```python
from build123d import *

# Parameters (mm, degrees)
F1_DEPTH = 91.42907
F2_R     = 7.5
F3_DEPTH = 2
F4_DEPTH = 5.7
F5_R     = 5
F6_DEPTH = 25
F6_TAPER = 13
F7_SIZE  = 0.5


with BuildPart() as f1:
    # F0 (on Top) → F1 (new body)
    with BuildSketch(Plane.XY):
        Polygon((1, 6.5773502692), (-1, 6.5773502692), (-1, 0.5773502692), (-6.1961524227, -2.4226497308), (-5.1961524227, -4.1547005384), (0, -1.1547005384), (5.1961524227, -4.1547005384), (6.1961524227, -2.4226497308), (1, 0.5773502692), align=None)
    extrude(amount=F1_DEPTH)

    # F2 (on face) → F3 (join)
    with BuildSketch(Plane.XY.offset(91.42907)):
        Circle(F2_R)
        with BuildLine():
            ThreePointArc((1, 5.941432908), (4.6003056964, 3.8907341852), (6.025, 0))
            ThreePointArc((6.025, 0), (5.9293486908, -1.0693217956), (5.6454318332, -2.1046910502))
            Line((5.6454318332, -2.1046910502), (6.1961524227, -2.4226497308))
            Line((6.1961524227, -2.4226497308), (5.1961524227, -4.1547005384))
            Line((5.1961524227, -4.1547005384), (4.6454318332, -3.8367418578))
            ThreePointArc((4.6454318332, -3.8367418578), (0, -6.025), (-4.6454318332, -3.8367418578))
            Line((-4.6454318332, -3.8367418578), (-5.1961524227, -4.1547005384))
            Line((-5.1961524227, -4.1547005384), (-6.1961524227, -2.4226497308))
            Line((-6.1961524227, -2.4226497308), (-5.6454318332, -2.1046910502))
            ThreePointArc((-5.6454318332, -2.1046910502), (-5.2178030578, 3.0125), (-1, 5.941432908))
            Line((-1, 5.941432908), (-1, 6.5773502692))
            Line((-1, 6.5773502692), (1, 6.5773502692))
            Line((1, 6.5773502692), (1, 5.941432908))
        make_face(mode=Mode.SUBTRACT)
        with BuildLine():
            Line((1, 0.5773502692), (1, 5.941432908))
            ThreePointArc((1, 5.941432908), (0, 6.025), (-1, 5.941432908))
            Line((-1, 5.941432908), (-1, 0.5773502692))
            Line((-1, 0.5773502692), (-5.6454318332, -2.1046910502))
            ThreePointArc((-5.6454318332, -2.1046910502), (-5.2178030578, -3.0125), (-4.6454318332, -3.8367418578))
            Line((-4.6454318332, -3.8367418578), (0, -1.1547005384))
            Line((0, -1.1547005384), (4.6454318332, -3.8367418578))
            ThreePointArc((4.6454318332, -3.8367418578), (5.2178030578, -3.0125), (5.6454318332, -2.1046910502))
            Line((5.6454318332, -2.1046910502), (1, 0.5773502692))
        make_face()
        with BuildLine():
            ThreePointArc((5.6454318332, -2.1046910502), (5.9293486908, -1.0693217956), (6.025, 0))
            ThreePointArc((6.025, 0), (4.6003056964, 3.8907341852), (1, 5.941432908))
            Line((1, 5.941432908), (1, 0.5773502692))
            Line((1, 0.5773502692), (5.6454318332, -2.1046910502))
        make_face()
        with BuildLine():
            ThreePointArc((-4.6454318332, -3.8367418578), (0, -6.025), (4.6454318332, -3.8367418578))
            Line((4.6454318332, -3.8367418578), (0, -1.1547005384))
            Line((0, -1.1547005384), (-4.6454318332, -3.8367418578))
        make_face()
        with BuildLine():
            Line((-1, 0.5773502692), (-1, 5.941432908))
            ThreePointArc((-1, 5.941432908), (-5.2178030578, 3.0125), (-5.6454318332, -2.1046910502))
            Line((-5.6454318332, -2.1046910502), (-1, 0.5773502692))
        make_face()
        with BuildLine():
            ThreePointArc((-4.6454318332, -3.8367418578), (-5.2178030578, -3.0125), (-5.6454318332, -2.1046910502))
            Line((-5.6454318332, -2.1046910502), (-6.1961524227, -2.4226497308))
            Line((-6.1961524227, -2.4226497308), (-5.1961524227, -4.1547005384))
            Line((-5.1961524227, -4.1547005384), (-4.6454318332, -3.8367418578))
        make_face()
        with BuildLine():
            Line((6.1961524227, -2.4226497308), (5.6454318332, -2.1046910502))
            ThreePointArc((5.6454318332, -2.1046910502), (5.2178030578, -3.0125), (4.6454318332, -3.8367418578))
            Line((4.6454318332, -3.8367418578), (5.1961524227, -4.1547005384))
            Line((5.1961524227, -4.1547005384), (6.1961524227, -2.4226497308))
        make_face()
        with BuildLine():
            ThreePointArc((-1, 5.941432908), (0, 6.025), (1, 5.941432908))
            Line((1, 5.941432908), (1, 6.5773502692))
            Line((1, 6.5773502692), (-1, 6.5773502692))
            Line((-1, 6.5773502692), (-1, 5.941432908))
        make_face()
    extrude(amount=F3_DEPTH)

    # F2 (on face) → F4 (join)
    with BuildSketch(Plane.XY.offset(91.42907)):
        Circle(F2_R)
        with BuildLine():
            ThreePointArc((1, 5.941432908), (4.6003056964, 3.8907341852), (6.025, 0))
            ThreePointArc((6.025, 0), (5.9293486908, -1.0693217956), (5.6454318332, -2.1046910502))
            Line((5.6454318332, -2.1046910502), (6.1961524227, -2.4226497308))
            Line((6.1961524227, -2.4226497308), (5.1961524227, -4.1547005384))
            Line((5.1961524227, -4.1547005384), (4.6454318332, -3.8367418578))
            ThreePointArc((4.6454318332, -3.8367418578), (0, -6.025), (-4.6454318332, -3.8367418578))
            Line((-4.6454318332, -3.8367418578), (-5.1961524227, -4.1547005384))
            Line((-5.1961524227, -4.1547005384), (-6.1961524227, -2.4226497308))
            Line((-6.1961524227, -2.4226497308), (-5.6454318332, -2.1046910502))
            ThreePointArc((-5.6454318332, -2.1046910502), (-5.2178030578, 3.0125), (-1, 5.941432908))
            Line((-1, 5.941432908), (-1, 6.5773502692))
            Line((-1, 6.5773502692), (1, 6.5773502692))
            Line((1, 6.5773502692), (1, 5.941432908))
        make_face(mode=Mode.SUBTRACT)
    extrude(amount=F4_DEPTH)

    # F5
    f5_edges = [f1.edges().sort_by_distance(p)[0] for p in [
        (-1, 0.57735, 45.714535),
        (1, 0.57735, 45.714535),
        (0, -1.154701, 45.714535),
    ]]
    fillet(f5_edges, radius=F5_R)

    # F2 (on face) → F6 (join)
    with BuildSketch(Plane.XY.offset(91.42907)):
        Circle(F2_R)
        with BuildLine():
            ThreePointArc((1, 5.941432908), (4.6003056964, 3.8907341852), (6.025, 0))
            ThreePointArc((6.025, 0), (5.9293486908, -1.0693217956), (5.6454318332, -2.1046910502))
            Line((5.6454318332, -2.1046910502), (6.1961524227, -2.4226497308))
            Line((6.1961524227, -2.4226497308), (5.1961524227, -4.1547005384))
            Line((5.1961524227, -4.1547005384), (4.6454318332, -3.8367418578))
            ThreePointArc((4.6454318332, -3.8367418578), (0, -6.025), (-4.6454318332, -3.8367418578))
            Line((-4.6454318332, -3.8367418578), (-5.1961524227, -4.1547005384))
            Line((-5.1961524227, -4.1547005384), (-6.1961524227, -2.4226497308))
            Line((-6.1961524227, -2.4226497308), (-5.6454318332, -2.1046910502))
            ThreePointArc((-5.6454318332, -2.1046910502), (-5.2178030578, 3.0125), (-1, 5.941432908))
            Line((-1, 5.941432908), (-1, 6.5773502692))
            Line((-1, 6.5773502692), (1, 6.5773502692))
            Line((1, 6.5773502692), (1, 5.941432908))
        make_face(mode=Mode.SUBTRACT)
        with BuildLine():
            ThreePointArc((-4.6454318332, -3.8367418578), (-5.2178030578, -3.0125), (-5.6454318332, -2.1046910502))
            Line((-5.6454318332, -2.1046910502), (-6.1961524227, -2.4226497308))
            Line((-6.1961524227, -2.4226497308), (-5.1961524227, -4.1547005384))
            Line((-5.1961524227, -4.1547005384), (-4.6454318332, -3.8367418578))
        make_face()
        with BuildLine():
            Line((-1, 0.5773502692), (-1, 5.941432908))
            ThreePointArc((-1, 5.941432908), (-5.2178030578, 3.0125), (-5.6454318332, -2.1046910502))
            Line((-5.6454318332, -2.1046910502), (-1, 0.5773502692))
        make_face()
        with BuildLine():
            Line((1, 0.5773502692), (1, 5.941432908))
            ThreePointArc((1, 5.941432908), (0, 6.025), (-1, 5.941432908))
            Line((-1, 5.941432908), (-1, 0.5773502692))
            Line((-1, 0.5773502692), (-5.6454318332, -2.1046910502))
            ThreePointArc((-5.6454318332, -2.1046910502), (-5.2178030578, -3.0125), (-4.6454318332, -3.8367418578))
            Line((-4.6454318332, -3.8367418578), (0, -1.1547005384))
            Line((0, -1.1547005384), (4.6454318332, -3.8367418578))
            ThreePointArc((4.6454318332, -3.8367418578), (5.2178030578, -3.0125), (5.6454318332, -2.1046910502))
            Line((5.6454318332, -2.1046910502), (1, 0.5773502692))
        make_face()
        with BuildLine():
            ThreePointArc((-4.6454318332, -3.8367418578), (0, -6.025), (4.6454318332, -3.8367418578))
            Line((4.6454318332, -3.8367418578), (0, -1.1547005384))
            Line((0, -1.1547005384), (-4.6454318332, -3.8367418578))
        make_face()
        with BuildLine():
            ThreePointArc((5.6454318332, -2.1046910502), (5.9293486908, -1.0693217956), (6.025, 0))
            ThreePointArc((6.025, 0), (4.6003056964, 3.8907341852), (1, 5.941432908))
            Line((1, 5.941432908), (1, 0.5773502692))
            Line((1, 0.5773502692), (5.6454318332, -2.1046910502))
        make_face()
        with BuildLine():
            Line((6.1961524227, -2.4226497308), (5.6454318332, -2.1046910502))
            ThreePointArc((5.6454318332, -2.1046910502), (5.2178030578, -3.0125), (4.6454318332, -3.8367418578))
            Line((4.6454318332, -3.8367418578), (5.1961524227, -4.1547005384))
            Line((5.1961524227, -4.1547005384), (6.1961524227, -2.4226497308))
        make_face()
        with BuildLine():
            ThreePointArc((-1, 5.941432908), (0, 6.025), (1, 5.941432908))
            Line((1, 5.941432908), (1, 6.5773502692))
            Line((1, 6.5773502692), (-1, 6.5773502692))
            Line((-1, 6.5773502692), (-1, 5.941432908))
        make_face()
    extrude(amount=-F6_DEPTH, taper=F6_TAPER)

    # F7
    f7_edges = [f1.edges().sort_by_distance(p)[0] for p in [
        (-6.196152, -2.42265, 43.880013),
        (-1, 6.57735, 43.880013),
        (1, 6.57735, 43.880013),
        (6.196152, -2.42265, 43.880013),
        (5.196152, -4.154701, 43.880013),
        (-5.196152, -4.154701, 43.880013),
    ]]
    chamfer(f7_edges, length=F7_SIZE)

    # F8: F1 across plane


with BuildPart() as f1_1:
    add(f1.part)
    add(f1.part.mirror(Plane.XY))


solid = f1_1.part
```
The model under review builds one solid part; all positions refer to its coordinate system, in mm. A direction names the side the tool comes from. Round coordinates to 2 decimals unless told otherwise and drop trailing zeros. Order: outer loops, then holes, each group sorted by start corner. A loop starts at its lowest first (then second) coordinate and runs counter-clockwise, first axis right, second up. Notation, with made-up numbers: (34.25, 4) - (69.25, 4) arc R32 cw to (69.25, 42) - close; hole circle Ø4 at (10.25, 75.25). An arc over 180 degrees is marked (long way). Answer in a Markdown table with one row per item.
(1) Machinability: for faces 5 (the face through (-5.255, 2.948, 95.253)), 6 (the face through (-6, 2, 97.129)), 7 (the face through (-5.255, 2.948, -95.253)), 8 (the face through (-0.04, -1.93, -1.04)), 9 (the face through (2.157, -4.147, 79.188)), which of the approach directions +Z, -Z, +X, -X, +Y, -Y give a long, thin tool a straight path to every point of the face, cutting with its end or side? Answer none if there is none.
Result set:
| item | result |
|---|---|
| face 5 | +Z |
| face 6 | +Z, +X, -X, +Y, -Y |
| face 7 | -Z |
| face 8 | -Y |
| face 9 | none |
(2) Mouldability with a two-part tool opening along Y and no side actions: class faces 1 (the face through (-6, 2, -97.129)), 2 (the face through (0.074, -6.025, -95.253)), 3 (the face through (0, 0, -93.429)), 4 (the face through (-7.493, 0.33, -94.239)) as released by +Y, released by -Y, zero draft, split by the parting line, or undercut.
Result set:
| item | result |
|---|---|
| face 1 | zero draft |
| face 2 | undercut |
| face 3 | undercut |
| face 4 | split by the parting line |
(3) Take a section at A-A on z = -16. Write out the cut boundary in (x, y).
Result set:
| item | result |
|---|---|
| outline | (-5.95, -2.86) - (-5.45, -3.72) - (-4.76, -3.9) - (-2.5, -2.6) arc R5 cw to (2.5, -2.6) - (4.76, -3.9) - (5.45, -3.72) - (5.95, -2.86) - (5.76, -2.17) - (3.5, -0.87) arc R5 cw to (1, 3.46) - (1, 6.08) - (0.5, 6.58) - (-0.5, 6.58) - (-1, 6.08) - (-1, 3.46) arc R5 cw to (-3.5, -0.87) - (-5.76, -2.17) - close |
(4) For line 1 (Z direction, x = 0.25, y = 0.75); line 2 (X direction, y = 3.75, z = -20.5); line 3 (X direction, y = 6.5, z = 83.5), list the stretches that pass through material, from the lowest coordinate up. Write a range as from..to.
Result set:
| item | result |
|---|---|
| line 1 | z = -93.43..93.43 |
| line 2 | x = -1..1 |
| line 3 | x = -0.58..0.58 |
(5) Clearance check with flat-ended pins moving along their axes: P1, Ø5, axis at x = -1.5, z = -29.5, coming from the +Y side; P2, Ø8, axis at y = 4.5, z = -61.5, coming from the -X side; P3, Ø0.5, axis at y = 6.5, z = 95.5, coming from the +X side; P4, Ø2, axis at y = -6, z = -69, coming from the +X side. State where each tip first meets the part, or that it passes through.
Result set:
| item | result |
|---|---|
| P1 | stops at y = 6.58 |
| P2 | stops at x = -1.97 |
| P3 | stops at x = 4.15 |
| P4 | passes through |
